Work out the finished part from the listing and answer in its coordinate system (mm). A direction names the side the tool comes from. Coordinates: 2 decimals unless noted, no trailing zeros. Order: outer loops, then holes, each group sorted by start corner. A loop starts at its lowest first (then second) coordinate and runs counter-clockwise, first axis right, second up. Notation, with made-up numbers: (64, 12) -> (74, 12) arc R22 cw to (74, 25) -> close; hole circle Ø7 at (-4.5, -23.75). An arc over 180 degrees is marked (long way). Write item = value, one per line. Start each with the question number.
Q1. For a pull along X with two mould halves and no side action, classify faces 4 (the cylindrical face through (95.98, 0.84, 4.26)), 5 (the flat face through (38, 1.7, 3)), 6 (the flat face through (103.05, 0.84, 14.88)) as +X half, -X half, draft (parallel to the pull), parting line (faces both ways), or undercut.
Q2. The part is cut by section B-B, the plane z = 7.5. Determine the outline of the cut face in (x, y).
Q3. The part is cut by section C-C, the plane y = 1.15. Determine the outline of the cut face in (x, z).
Q4. Straight lines are drawn through the part: L1, parallel to X at y = 0.8, z = 3.5; L2, parallel to Z at x = 83.5, y = 0.7; L3, parallel to X at y = 1.65, z = 10. For each, find the intervals that lie inside material, in ascending order. Write a range as from..to.
Q5. The part is cut by section A-A, the plane x = 86. Determine the outline of the cut face in (y, z), plus the area to 3 significant figures.
Q6. Which of the six approach directions +Z, -Z, +X, -X, +Y, -Y give full straight-line access (tool end or side, diameter ignored) to faces 1 (the cylindrical face through (65.983, 0.838, 3.848)), 2 (the flat face through (38, 0, 3)), 3 (the flat face through (38.373, 0.838, 15.364))?
Q7. The part is cut by section D-D, the plane z = -3.5. Determine the outline of the cut face in (x, y), plus the area to 3 significant figures.
```python
from build123d import *

# Parameters (mm, degrees)
BOSS_EXTRUDE1_DEPTH = 1.7


with BuildPart() as part:
    # Sketch1 → Boss-Extrude1 (new body)
    with BuildSketch(Plane(origin=(0, 0, 0), x_dir=(1, 0, 0), z_dir=(0, 1, 0))):
        Polygon((-8.017928363, -16.55461165), (-8.017928363, -1.55461165), (1.182071637, -1.55461165), (1.182071637, -19.55461165), (34.182071637, -19.55461165), (42.682071637, -11.05461165), (60.682071637, -11.05461165), (69.503836167, -20.05461165), (97.769928994, -20.05461165), (108.482071637, -9.55461165), (108.482071637, 13.94538835), (-31.517928363, 13.94538835), (-31.517928363, -16.55461165), align=None)
        with BuildLine():
            ThreePointArc((72.690509661, 8.44538835), (65.982071637, -4.05461165), (72.690509661, -16.55461165))
            Line((72.690509661, -16.55461165), (89.273633613, -16.55461165))
            ThreePointArc((89.273633613, -16.55461165), (95.982071637, -4.05461165), (89.273633613, 8.44538835))
            Line((89.273633613, 8.44538835), (72.690509661, 8.44538835))
        make_face(mode=Mode.SUBTRACT)
    extrude(amount=BOSS_EXTRUDE1_DEPTH)


solid = part.part
```
Model answer:
q1.face_4 = undercut
q1.face_5 = draft
q1.face_6 = +X half
q2.outline = (-31.52, 0) -> (-8.02, 0) -> (-8.02, 1.7) -> (-31.52, 1.7) -> close; (1.18, 0) -> (66.38, 0) -> (66.38, 1.7) -> (1.18, 1.7) -> close; (95.58, 0) -> (108.48, 0) -> (108.48, 1.7) -> (95.58, 1.7) -> close
q3.outline = (-31.52, -13.95) -> (108.48, -13.95) -> (108.48, 9.55) -> (97.77, 20.05) -> (69.5, 20.05) -> (60.68, 11.05) -> (42.68, 11.05) -> (34.18, 19.55) -> (1.18, 19.55) -> (1.18, 1.55) -> (-8.02, 1.55) -> (-8.02, 16.55) -> (-31.52, 16.55) -> close; hole (72.69, -8.45) -> (89.27, -8.45) arc R15 ccw to (89.27, 16.55) -> (72.69, 16.55) arc R15 ccw to start
q4.L1 = -31.52..-8.02, 1.18..65.99, 95.97..108.48
q4.L2 = -13.95..-8.45, 16.55..20.05
q4.L3 = -31.52..-8.02, 1.18..67.21, 94.75..108.03
q5.outline = (0, -13.95) -> (1.7, -13.95) -> (1.7, -8.45) -> (0, -8.45) -> close; (0, 16.55) -> (1.7, 16.55) -> (1.7, 20.05) -> (0, 20.05) -> close
q5.area = 15.3 mm2
q6.face_1 = +Y, -Y
q6.face_2 = +Z, -Z, +X, -X, -Y
q6.face_3 = +Z, +Y, -Y
q7.outline = (-31.52, 0) -> (68.02, 0) -> (68.02, 1.7) -> (-31.52, 1.7) -> close; (93.94, 0) -> (108.48, 0) -> (108.48, 1.7) -> (93.94, 1.7) -> close
q7.area = 194 mm2
